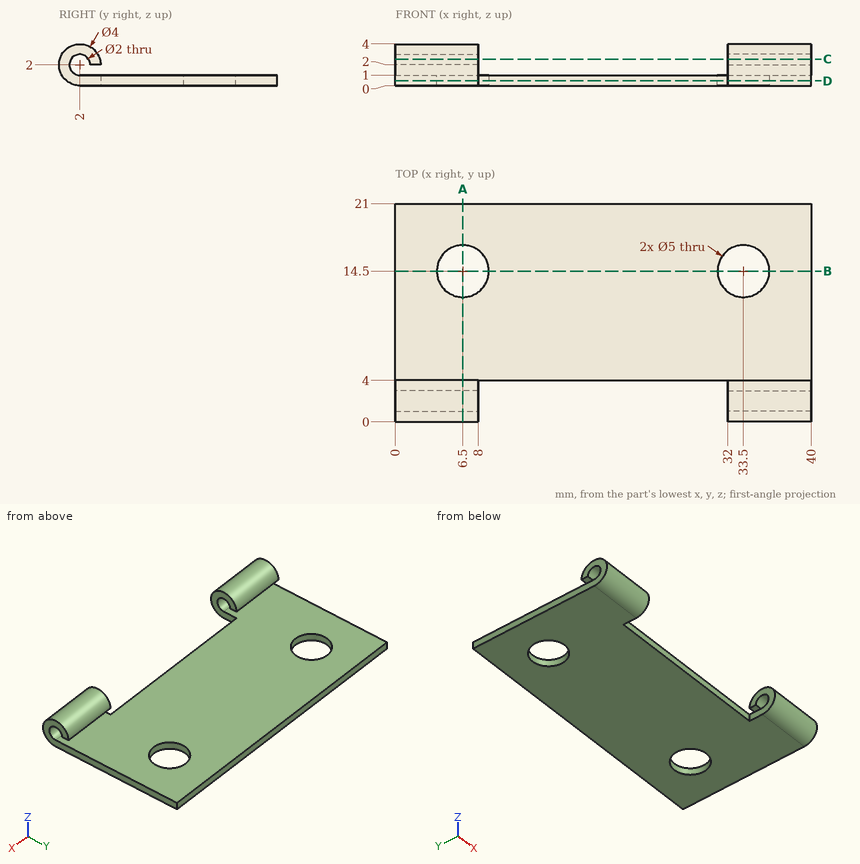
Here's the drawing with two shaded views (mm, measured from the low corner). I have some questions. Coordinates: 2 decimals unless noted, no trailing zeros. Write each loop counter-clockwise with the first axis right and the second up, starting at its lowest first coordinate (ties: lowest second). Pieces come first, ordered by that corner, then holes.
Item 1: Will these pins go through, and if not, where does the flat tip stop? pin 1 (9.5 mm diameter, centred on x = 21.5, y = 12.5, fed in from +Z); pin 2 (1.8 mm diameter, centred on y = 2, z = 2, fed in from -X); pin 3 (1 mm diameter, centred on x = 30.5, z = 0.5, fed in from -Y).
Item 2: I want a section at B-B on y = 14.5. Write out the boundary of the cut face in (x, z), and give its area (3 significant figures).
Item 3: I want a section at A-A on x = 6.5. Write out the boundary of the cut face in (y, z), and give its area (3 significant figures).
Item 4: I want a section at C-C on z = 2.55. Write out the boundary of the cut face in (x, y).
Item 5: I want a section at D-D on z = 0.45. Write out the boundary of the cut face in (x, y).
Item 6: If I drill on line 1 (X direction, y = 2, z = 3.35); line 2 (Z direction, x = 5.5, y = 2); line 3 (Z direction, x = 3.5, y = 15.75), over which ranges is the centre line in solid material (lowest first)?
Findings below:
1. pin 1: stops at z = 1
1. pin 2: passes through
1. pin 3: stops at y = 4
2. outline: (0, 0) - (4, 0) - (4, 1) - (0, 1) - close; (9, 0) - (31, 0) - (31, 1) - (9, 1) - close; (36, 0) - (40, 0) - (40, 1) - (36, 1) - close
2. area: 30.0 mm2
3. outline: (2, 0) - (12, 0) - (12, 1) - (2, 1) arc R1 cw (long way) to (3, 2) - (4, 2) arc R2 ccw (long way) to start; (17, 0) - (21, 0) - (21, 1) - (17, 1) - close
3. area: 21.1 mm2
4. outline: (0, 0.08) - (8, 0.08) - (8, 1.16) - (0, 1.16) - close; (0, 2.84) - (8, 2.84) - (8, 3.92) - (0, 3.92) - close; (32, 0.08) - (40, 0.08) - (40, 1.16) - (32, 1.16) - close; (32, 2.84) - (40, 2.84) - (40, 3.92) - (32, 3.92) - close
5. outline: (0, 0.74) - (8, 0.74) - (8, 4) - (32, 4) - (32, 0.74) - (40, 0.74) - (40, 21) - (0, 21) - close; hole circle Ø5 at (6.5, 14.5); hole circle Ø5 at (33.5, 14.5)
6. line 1: x = 0 to 8, 32 to 40
6. line 2: z = 0 to 1, 3 to 4
6. line 3: z = 0 to 1
